Autodesk Inventor part; units mm, degrees
ref_plane "YZ Plane" through (0, 0, 0) normal (1, 0, 0) x (0, 1, 0)
ref_plane "XZ Plane" through (0, 0, 0) normal (0, 1, 0) x (-1, 0, 0)
ref_plane "XY Plane" through (0, 0, 0) normal (0, 0, 1) x (1, 0, 0)
sketch "스케치1" plane through (0, 0, 0) normal (0, 0, 1) x (1, 0, 0)
  arc A0 (-6.843, 8.7398) -> (6.843, 8.7398) centre (0, 0) ccw
  circle A1 centre (0, -8) radius 1.05
  circle A2 centre (-5.6569, -5.6569) radius 1.05
  circle A3 centre (-8, 0) radius 1.05
  circle A4 centre (-5.6569, 5.6569) radius 1.05
  circle A5 centre (0, 8) radius 1.05
  circle A6 centre (5.6569, 5.6569) radius 1.05
  circle A7 centre (8, 0) radius 1.05
  circle A8 centre (5.6569, -5.6569) radius 1.05
  line L0 (-5.6569, 5.6569) -> (5.6569, 5.6569)
  line L1 (5.6569, 5.6569) -> (5.6569, 13.3625)
  line L2 (5.6569, 13.3625) -> (-5.6569, 13.3625)
  line L3 (-5.6569, 13.3625) -> (-5.6569, 5.6569)
  line L4 (-3.61, 0) -> (3.61, 0)
  line L5 (3.61, 13.6832) -> (-3.61, 13.6832)
  line L6 (11.1, 0) -> (11.1, -39)
  line L7 (-11.1, 0) -> (-11.1, -39)
  line L8 (-11.1, -39) -> (11.1, -39)
  circle A9 centre (8, 0) radius 1.15
  circle A10 centre (5.6569, -5.6569) radius 1.15
  circle A11 centre (5.6569, 5.6569) radius 1.15
  circle A12 centre (0, 8) radius 1.15
  circle A13 centre (0, -8) radius 1.15
  circle A14 centre (-5.6569, 5.6569) radius 1.15
  circle A15 centre (-8, 0) radius 1.15
  circle A16 centre (-5.6569, -5.6569) radius 1.15
  circle A17 centre (0, 0) radius 4.2
  arc A18 (-7.5626, 8.1251) -> (7.5626, 8.1251) centre (0, 0) ccw
  line L9 (4.2, 0) -> (-4.2, 0)
  line L10 (-4.2, 0) -> (-4.2, 6.6611)
  line L11 (-4.2, 14) -> (4.2, 14)
  line L12 (4.2, 6.6611) -> (4.2, 0)
  arc A19 (7.5626, 8.1251) -> (4.2, 6.6611) centre (6.2, 6.6611) ccw
  arc A20 (-4.2, 6.6611) -> (-7.5626, 8.1251) centre (-6.2, 6.6611) ccw
  point P0 (0, 0)
  point P1 (3.61, 10.4966)
  point P2 (-3.61, 10.4966)
  point P3 (5.6569, 6.7069)
  point P4 (4.6069, 5.6569)
  point P5 (-4.6069, 5.6569)
  point P6 (-5.6569, 6.7069)
  point P7 (-4.5069, 5.6569)
  point P8 (-5.6569, 6.8069)
  point P9 (5.6569, 6.8069)
  point P10 (4.5069, 5.6569)
  point P11 (4.2, 10.2747)
  point P12 (-4.2, 10.2747)
  point P13 (-7.5626, 8.1251)
  point P14 (7.5626, 8.1251)
  dimension "d0" = 22.2
  dimension "d5" = 0.1
  dimension "d6" = 0.1
  dimension "d7" = 0.1
  dimension "d8" = 0.1
  dimension "d9" = 0.1
  dimension "d10" = 0.1
  dimension "d11" = 0.1
  dimension "d12" = 0.1
  dimension "d23" = 2
extrude "돌출1" add sketch "스케치1" along normal blind 6 contours A20 L3 A14 L0 L10 A17 L12 A11 L1 A19 A0 | A0 L6 L8 L7 | A20 L10 L0 A14 L3 | L1 A11 L0 L12 A19
sketch "스케치2" plane through (0, 0, 6) normal (0, 0, 1) x (1, 0, 0)
  line L0 (11.1, -33) -> (11.1, -39)
  line L1 (11.1, -39) -> (-11.1, -39)
  line L2 (-11.1, -39) -> (-11.1, -33)
  line L3 (-11.1, -33) -> (11.1, -33)
  point P0 (0, 0)
extrude "돌출2" add sketch "스케치2" along normal blind 41
sketch "스케치3" plane through (0, 0, 47) normal (0, 0, 1) x (1, 0, 0)
  line L0 (-11.1, -33) -> (11.1, -33)
  arc A0 (-11.1, 0) -> (11.1, 0) centre (0, 0) ccw
  line L1 (-11.1, 0) -> (-11.1, -33)
  arc A1 (4.5069, 5.6569) -> (5.6569, 6.8069) centre (5.6569, 5.6569) ccw
  circle A2 centre (8, 0) radius 1.15
  circle A3 centre (5.6569, -5.6569) radius 1.15
  circle A4 centre (0, -8) radius 1.15
  circle A5 centre (-8, 0) radius 1.15
  circle A6 centre (-5.6569, -5.6569) radius 1.15
  arc A7 (-5.6569, 6.8069) -> (-4.5069, 5.6569) centre (-5.6569, 5.6569) ccw
  line L2 (11.1, -39) -> (11.1, -33)
  line L3 (-11.1, -33) -> (-11.1, -39)
  line L4 (11.1, -33) -> (-11.1, -33)
  line L5 (-11.1, -33) -> (-11.1, -39)
  line L6 (-11.1, -39) -> (11.1, -39)
  line L7 (11.1, -39) -> (11.1, -33)
  circle A8 centre (0, 0) radius 6
  arc A9 (-9.7582, 5.2902) -> (9.7582, 5.2902) centre (0, 0) ccw
  line L8 (6, 0) -> (-6, 0)
  line L9 (-6, 0) -> (-6, 4.337)
  line L10 (-6, 12) -> (6, 12)
  line L11 (6, 4.337) -> (6, 0)
  arc A10 (9.7582, 5.2902) -> (6, 4.337) centre (8, 4.337) ccw
  arc A11 (-6, 4.337) -> (-9.7582, 5.2902) centre (-8, 4.337) ccw
  line L12 (-11.1, -33) -> (11.1, -33)
  line L13 (11.1, -33) -> (11.1, 0)
  arc A12 (11.1, 0) -> (7.5626, 8.1251) centre (0, 0) ccw
  line L14 (-11.1, 0) -> (-11.1, -33)
  circle A13 centre (5.6569, 5.6569) radius 1.15
  circle A14 centre (-5.6569, 5.6569) radius 1.15
  arc A15 (7.5626, 8.1251) -> (4.2, 6.6611) centre (6.2, 6.6611) ccw
  line L15 (4.2, 6.6611) -> (4.2, 0)
  arc A16 (-4.2, 0) -> (4.2, 0) centre (0, 0) ccw
  line L16 (-4.2, 0) -> (-4.2, 6.6611)
  arc A17 (-4.2, 6.6611) -> (-7.5626, 8.1251) centre (-6.2, 6.6611) ccw
  arc A18 (-7.5626, 8.1251) -> (-11.1, 0) centre (0, 0) ccw
  point P0 (-6.843, 8.7398)
  point P1 (6, 9.3386)
  point P2 (-6, 9.3386)
  point P3 (6.7765, 5.9192)
  point P4 (6.0128, 4.5633)
  point P5 (-6.0128, 4.5633)
  point P6 (-6.7765, 5.9192)
  point P7 (-9.7582, 5.2902)
  point P8 (5.6569, 6.8069)
  point P9 (9.7582, 5.2902)
  point P10 (-9.7582, 5.2902)
  dimension "d21" = 2
extrude "돌출3" add sketch "스케치3" along normal blind 6 contours L1 A0 L13 L0 | L0 L2 L6 L3 | A9 A11 A7 L9 A8 L11 A10 A1 A0 | A18 A17 L16 A8 L9 A11 A7 A14 | A10 A1 A13 L11 A8 L15 A15 A12 | L16 L8 A8 | A8 L8 L15 | L8 A16 A8
sketch "스케치4" plane through (-11.1, -33, 6) normal (0, 1, 0) x (1, 0, 0)
  circle A0 centre (3.3218, -12.7218) radius 1.55
  circle A1 centre (3.3218, -28.2782) radius 1.55
  circle A2 centre (18.8782, -28.2782) radius 1.55
  circle A3 centre (18.8782, -12.7218) radius 1.55
  circle A4 centre (11.1, -20.5) radius 13.9
  circle A5 centre (22.1, -20.5) radius 1.55
  circle A6 centre (11.1, -31.5) radius 1.55
  circle A7 centre (0.1, -20.5) radius 1.55
  circle A8 centre (11.1, -9.5) radius 1.55
  circle A9 centre (11.1, -20.5) radius 5.2
  circle A10 centre (11.1, -20.5) radius 1.5
  circle A11 centre (11.1, -20.5) radius 13.9
  point P0 (11.1, 6)
extrude "돌출4" cut sketch "스케치4" against normal up to next contours A0 | A1 | A2 | A3 | A6 | A8 | A9 | A10
properties part number "arm_connect_3"
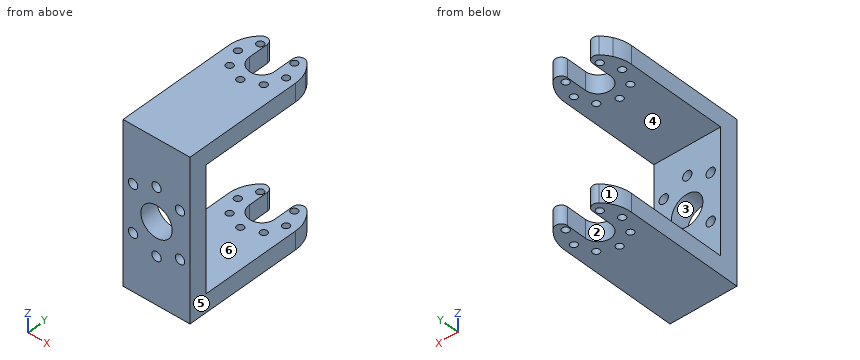
Verification items for the finished model (mm, model axes). Face numbers are marked on the shaded views. A direction names the side the tool comes from. Coordinates: 2 decimals unless noted, no trailing zeros. Loops run counter-clockwise (first coordinate to the right, second up) from the corner with the lowest first, then second, coordinate; pieces in that order, holes last. Notation, with made-up numbers: M -17.5,58.25 L 22.5,58.25 A33 ccw 22.5,86.25 Z; hole C 48,84.5 d10. An arc over 180 degrees is marked long. One line per item, written item: value.
1. Gauge pin test, flat ends, axial feed: P1, Ø6.5, axis at x = 5, z = 34, coming from the +Y side; P2, Ø5, axis at y = 3.5, z = 50.5, coming from the -X side. Record the tip position at first contact, or that the pin passes through.
Answers follow:
P1: y = -33
P2: x = -11.05
2. Material ranges on line 1 along Z through (x, y) = (-1.5, -14); line 2 along X through (y, z) = (0.5, 5); line 3 along Z through (x, y) = (-8, -34), recorded low to high. Write a range as from..to.
Answers follow:
line 1: 0..6, 47..53
line 2: -11.09..-9.04, -6.96..-4.2, 4.2..6.96, 9.04..11.09
line 3: 0..17.19, 20.26..32.74, 35.81..53
3. Mould release check, pull along X, two halves, no side actions. Record for the marked faces 1, 2, 3 and 4: pulls with the +X half, pulls with the -X half, needs draft (parallel to the pull), parting line crosses it, or undercut.
Answers follow:
face 1: pulls with the -X half
face 2: undercut
face 3: undercut
face 4: needs draft
4. Section check B-B on y = -21. Record the cut outline in (x, z).
Answers follow:
outline: M -11.1,0 L 11.1,0 L 11.1,6 L -11.1,6 Z; M -11.1,47 L 11.1,47 L 11.1,53 L -11.1,53 Z
5. Set-up check for the marked faces 5 and 6: record each of +Z, -Z, +X, -X, +Y, -Y from which the full face is reachable in a straight line by a thin tool's end or side.
Answers follow:
face 5: +Z, -Z, +X, +Y, -Y
face 6: +X, -X, +Y
6. Section check C-C on x = 0. Record the cut outline in (y, z), plus the area to 3 significant figures.
Answers follow:
outline: M -39,0 L -9.15,0 L -9.15,6 L -33,6 L -33,13.95 L -39,13.95 Z; M -39,17.05 L -33,17.05 L -33,21.3 L -39,21.3 Z; M -39,31.7 L -33,31.7 L -33,35.95 L -39,35.95 Z; M -39,39.05 L -33,39.05 L -33,47 L -9.15,47 L -9.15,53 L -39,53 Z; M -6.85,0 L -4.2,0 L -4.2,6 L -6.85,6 Z; M -6.85,47 L -4.2,47 L -4.2,53 L -6.85,53 Z
area: 536 mm^2
7. Section check A-A on z = 15.5. Record the cut outline in (x, y), plus the area to 3 significant figures.
Answers follow:
outline: M -11.1,-39 L -1.55,-39 L -1.55,-33 L -11.1,-33 Z; M 1.55,-39 L 11.1,-39 L 11.1,-33 L 1.55,-33 Z
area: 115 mm^2
